The listing builds one solid part. Answer for the finished solid, in the listing's coordinates (mm). Round coordinates to 2 decimals unless told otherwise and drop trailing zeros. Write each loop counter-clockwise with the first axis right and the second up, starting at its lowest first coordinate (ties: lowest second). Pieces come first, ordered by that corner, then holes. Notation, with made-up numbers: M 69.5,33 L 114.5,33 A22 ccw 114.5,71 Z; hole C -28,7 d1. An arc over 180 degrees is marked long. One line per item, written item: value. Start each with the question number.
(1) Section B-B (x = 150.1) is taken. Determine the outline of the cut face in (y, z).
(2) Given P1, Ø3, axis at x = 87.5, z = -220, coming from the +Y side; P2, Ø1, axis at x = 38.5, y = 3, coming from the -Z side; P3, Ø1.9, axis at x = 34.5, z = 3, coming from the -Y side; P4, Ø4, axis at x = 17.53, z = -54.65, coming from the -Y side, each flat-ended and moving along its own axis, determine where each tip first touches the part or whether it passes through.
(3) Section A-A (z = -31) is taken. Determine the outline of the cut face in (x, y), plus the area to 3 significant figures.
(4) Section D-D (y = 2.5) is taken. State how many separate pieces and enclosed holes the cut face has, plus the area to 3 significant figures.
(5) Section C-C (z = -158.15) is taken. Determine the outline of the cut face in (x, y), plus the area to 3 significant figures.
(6) Consider probe 1 along Z at (x, y) = (167.15, 2.75); probe 2 along Z at (x, y) = (150.1, 2.75); probe 3 along Z at (x, y) = (147.5, 2.5). Determine where each line is inside the solid, lowest interval first.
```python
from build123d import *

# Parameters (mm, degrees)
SKETCH4_W           = 184.15
SKETCH4_H           = 215.9
BOSS_EXTRUDE2_DEPTH = 6.35
BOSS_EXTRUDE3_DEPTH = 6.35
BOSS_EXTRUDE4_DEPTH = 6.35
SKETCH7_W           = 5.08
SKETCH7_H           = 6.35
BOSS_EXTRUDE5_DEPTH = 3.81
SKETCH12_R          = 2.54
CUT_EXTRUDE4_DEPTH  = 7.35
SKETCH18_R          = 2.5
CUT_EXTRUDE8_DEPTH  = 10
SKETCH19_R          = 2.5
CUT_EXTRUDE9_DEPTH  = 10
SKETCH20_R          = 3
CUT_EXTRUDE10_DEPTH = 7.35
CUT_EXTRUDE11_DEPTH = 6.35
CUT_EXTRUDE12_DEPTH = 6.35
CUT_EXTRUDE13_DEPTH = 6.35
CUT_EXTRUDE14_DEPTH = 6.35
CUT_EXTRUDE15_DEPTH = 6.35


with BuildPart() as part:
    # Sketch4 → Boss-Extrude2 (new body)
    with BuildSketch(Plane(origin=(0, 0, 0), x_dir=(1, 0, 0), z_dir=(0, 1, 0))):
        with Locations((92.075, 107.95)):
            Rectangle(SKETCH4_W, SKETCH4_H)
    extrude(amount=BOSS_EXTRUDE2_DEPTH)

    # Sketch5 → Boss-Extrude3 (add)
    with BuildSketch(Plane.XY):
        with BuildLine():
            Line((15.875, 6.35), (66.675, 6.35))
            ThreePointArc((66.675, 6.35), (69.85, 3.175), (66.675, 0))
            Line((66.675, 0), (15.875, 0))
            ThreePointArc((15.875, 0), (12.7, 3.175), (15.875, 6.35))
        make_face()
    boss_extrude3 = extrude(amount=BOSS_EXTRUDE3_DEPTH)

    # Mirror1: Boss-Extrude3 across plane
    add(boss_extrude3.mirror(Plane(origin=(92.075, 0, 0), x_dir=(0, 0, 1), z_dir=(1, 0, 0))))

    # Sketch6 → Boss-Extrude4 (add)
    with BuildSketch(Plane(origin=(0, 0, -215.9), x_dir=(-1, 0, 0), z_dir=(0, 0, -1))):
        with BuildLine():
            Line((-117.475, 6.35), (-66.675, 6.35))
            ThreePointArc((-66.675, 6.35), (-63.5, 3.175), (-66.675, 0))
            Line((-66.675, 0), (-117.475, 0))
            ThreePointArc((-117.475, 0), (-120.65, 3.175), (-117.475, 6.35))
        make_face()
        with BuildLine():
            Line((-28.575, 6.35), (-3.175, 6.35))
            ThreePointArc((-3.175, 6.35), (0, 3.175), (-3.175, 0))
            Line((-3.175, 0), (-28.575, 0))
            ThreePointArc((-28.575, 0), (-31.75, 3.175), (-28.575, 6.35))
        make_face()
        with BuildLine():
            Line((-155.575, 6.35), (-180.975, 6.35))
            ThreePointArc((-180.975, 6.35), (-184.15, 3.175), (-180.975, 0))
            Line((-180.975, 0), (-155.575, 0))
            ThreePointArc((-155.575, 0), (-152.4, 3.175), (-155.575, 6.35))
        make_face()
    extrude(amount=BOSS_EXTRUDE4_DEPTH)

    # Sketch7 → Boss-Extrude5 (add)
    with BuildSketch(Plane(origin=(184.15, 0, 0), x_dir=(0, 0, -1), z_dir=(1, 0, 0))):
        with Locations((100.33, 3.175)):
            Rectangle(SKETCH7_W, SKETCH7_H)
    boss_extrude5 = extrude(amount=BOSS_EXTRUDE5_DEPTH)

    # Mirror3: Boss-Extrude5 across plane
    add(boss_extrude5.mirror(Plane.ZY.offset(-92.075)))

    # Sketch12 → Cut-Extrude4 (cut, through all)
    with BuildSketch(Plane.XZ):
        with Locations((17.528627724, -54.65)):
            Circle(SKETCH12_R)
        with Locations((167.15, -54.65)):
            Circle(SKETCH12_R)
        with Locations((167.15, -106.15)):
            Circle(SKETCH12_R)
        with Locations((17.528627724, -106.15)):
            Circle(SKETCH12_R)
        with Locations((17.528627724, -158.15)):
            Circle(SKETCH12_R)
        with Locations((167.15, -158.15)):
            Circle(SKETCH12_R)
    extrude(amount=-CUT_EXTRUDE4_DEPTH, mode=Mode.SUBTRACT)

    # Sketch18 → Cut-Extrude8 (cut)
    with BuildSketch(Plane(origin=(0, 6.35, 0), x_dir=(1, 0, 0), z_dir=(0, 1, 0))):
        with Locations((105.290220108, 49.015069715)):
            Circle(SKETCH18_R)
        with Locations((133.990220108, 49.015069715)):
            Circle(SKETCH18_R)
        with Locations((119.640220108, 96.915069715)):
            Circle(SKETCH18_R)
    extrude(amount=-CUT_EXTRUDE8_DEPTH, mode=Mode.SUBTRACT)

    # Sketch19 → Cut-Extrude9 (cut)
    with BuildSketch(Plane(origin=(0, 6.35, 0), x_dir=(1, 0, 0), z_dir=(0, 1, 0))):
        with Locations((75.754890742, 56.124247339)):
            Circle(SKETCH19_R)
        with Locations((38.754890742, 56.124247339)):
            Circle(SKETCH19_R)
        with Locations((75.754890742, 93.124247339)):
            Circle(SKETCH19_R)
        with Locations((38.754890742, 93.124247339)):
            Circle(SKETCH19_R)
    extrude(amount=-CUT_EXTRUDE9_DEPTH, mode=Mode.SUBTRACT)

    # Sketch20 → Cut-Extrude10 (cut, through all)
    with BuildSketch(Plane.XZ):
        with Locations((150.1, -182.048287602)):
            Circle(SKETCH20_R)
        with Locations((34.1, -182.048287602)):
            Circle(SKETCH20_R)
        with Locations((150.1, -31)):
            Circle(SKETCH20_R)
        with Locations((34.1, -31)):
            Circle(SKETCH20_R)
    extrude(amount=-CUT_EXTRUDE10_DEPTH, mode=Mode.SUBTRACT)

    # Sketch21 → Cut-Extrude11 (cut)
    with BuildSketch(Plane(origin=(0, 0, -222.25), x_dir=(-1, 0, 0), z_dir=(0, 0, -1))):
        with BuildLine():
            Line((-155.575, 6.35), (-180.975, 6.35))
            ThreePointArc((-180.975, 6.35), (-184.15, 3.175), (-180.975, 0))
            Line((-180.975, 0), (-155.575, 0))
            ThreePointArc((-155.575, 0), (-152.4, 3.175), (-155.575, 6.35))
        make_face()
        with BuildLine():
            Line((-155.575, 6.25), (-180.975, 6.25))
            ThreePointArc((-180.975, 6.25), (-184.05, 3.175), (-180.975, 0.1))
            Line((-180.975, 0.1), (-155.575, 0.1))
            ThreePointArc((-155.575, 0.1), (-152.5, 3.175), (-155.575, 6.25))
        make_face(mode=Mode.SUBTRACT)
    extrude(amount=-CUT_EXTRUDE11_DEPTH, mode=Mode.SUBTRACT)

    # Sketch22 → Cut-Extrude12 (cut)
    with BuildSketch(Plane(origin=(0, 0, -222.25), x_dir=(-1, 0, 0), z_dir=(0, 0, -1))):
        with BuildLine():
            Line((-66.675, 6.35), (-117.475, 6.35))
            ThreePointArc((-117.475, 6.35), (-120.65, 3.175), (-117.475, 0))
            Line((-117.475, 0), (-66.675, 0))
            ThreePointArc((-66.675, 0), (-63.5, 3.175), (-66.675, 6.35))
        make_face()
        with BuildLine():
            Line((-66.675, 6.25), (-117.475, 6.25))
            ThreePointArc((-117.475, 6.25), (-120.55, 3.175), (-117.475, 0.1))
            Line((-117.475, 0.1), (-66.675, 0.1))
            ThreePointArc((-66.675, 0.1), (-63.6, 3.175), (-66.675, 6.25))
        make_face(mode=Mode.SUBTRACT)
    extrude(amount=-CUT_EXTRUDE12_DEPTH, mode=Mode.SUBTRACT)

    # Sketch23 → Cut-Extrude13 (cut)
    with BuildSketch(Plane(origin=(0, 0, -222.25), x_dir=(-1, 0, 0), z_dir=(0, 0, -1))):
        with BuildLine():
            Line((-28.575, 0), (-3.175, 0))
            ThreePointArc((-3.175, 0), (0, 3.175), (-3.175, 6.35))
            Line((-3.175, 6.35), (-28.575, 6.35))
            ThreePointArc((-28.575, 6.35), (-31.75, 3.175), (-28.575, 0))
        make_face()
        with BuildLine():
            Line((-28.575, 0.1), (-3.175, 0.1))
            ThreePointArc((-3.175, 0.1), (-0.1, 3.175), (-3.175, 6.25))
            Line((-3.175, 6.25), (-28.575, 6.25))
            ThreePointArc((-28.575, 6.25), (-31.65, 3.175), (-28.575, 0.1))
        make_face(mode=Mode.SUBTRACT)
    extrude(amount=-CUT_EXTRUDE13_DEPTH, mode=Mode.SUBTRACT)

    # Sketch24 → Cut-Extrude14 (cut)
    with BuildSketch(Plane.XY.offset(6.35)):
        with BuildLine():
            Line((15.875, 0), (66.675, 0))
            ThreePointArc((66.675, 0), (69.85, 3.175), (66.675, 6.35))
            Line((66.675, 6.35), (15.875, 6.35))
            ThreePointArc((15.875, 6.35), (12.7, 3.175), (15.875, 0))
        make_face()
        with BuildLine():
            Line((15.875, 0.1), (66.675, 0.1))
            ThreePointArc((66.675, 0.1), (69.75, 3.175), (66.675, 6.25))
            Line((66.675, 6.25), (15.875, 6.25))
            ThreePointArc((15.875, 6.25), (12.8, 3.175), (15.875, 0.1))
        make_face(mode=Mode.SUBTRACT)
    extrude(amount=-CUT_EXTRUDE14_DEPTH, mode=Mode.SUBTRACT)

    # Sketch25 → Cut-Extrude15 (cut)
    with BuildSketch(Plane.XY.offset(6.35)):
        with BuildLine():
            Line((168.275, 6.35), (117.475, 6.35))
            ThreePointArc((117.475, 6.35), (114.3, 3.175), (117.475, 0))
            Line((117.475, 0), (168.275, 0))
            ThreePointArc((168.275, 0), (171.45, 3.175), (168.275, 6.35))
        make_face()
        with BuildLine():
            Line((168.275, 6.25), (117.475, 6.25))
            ThreePointArc((117.475, 6.25), (114.4, 3.175), (117.475, 0.1))
            Line((117.475, 0.1), (168.275, 0.1))
            ThreePointArc((168.275, 0.1), (171.35, 3.175), (168.275, 6.25))
        make_face(mode=Mode.SUBTRACT)
    extrude(amount=-CUT_EXTRUDE15_DEPTH, mode=Mode.SUBTRACT)


solid = part.part
```
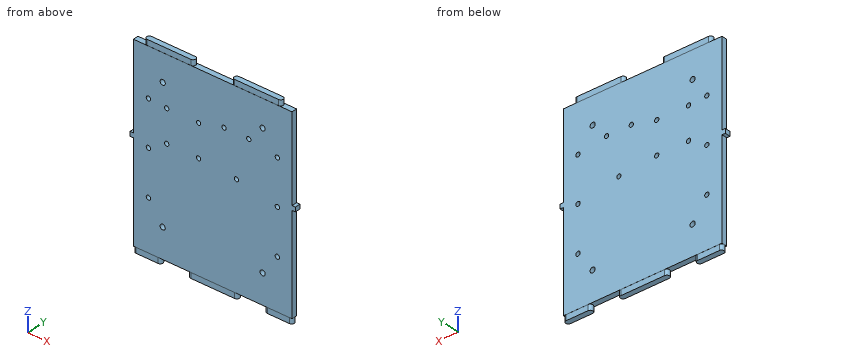
Recorded:
1. outline: M 0,-215.9 L 6.35,-215.9 L 6.35,-185.05 L 0,-185.05 Z; M 0,-179.05 L 6.35,-179.05 L 6.35,-34 L 0,-34 Z; M 0,-28 L 6.35,-28 L 6.35,0 L 6.25,0 L 6.25,6.35 L 0.1,6.35 L 0.1,0 L 0,0 Z
2. P1: stops at y = 6.25
2. P2: stops at z = -215.9
2. P3: stops at y = 0.1
2. P4: passes through
3. outline: M 0,0 L 31.1,0 L 31.1,6.35 L 0,6.35 Z; M 37.1,0 L 147.1,0 L 147.1,6.35 L 37.1,6.35 Z; M 153.1,0 L 184.15,0 L 184.15,6.35 L 153.1,6.35 Z
3. area: 1,090 mm2
4. separate pieces: 1
4. enclosed holes: 17
4. area: 40,900 mm2
5. outline: M 0,0 L 14.99,0 L 14.99,6.35 L 0,6.35 Z; M 20.07,0 L 164.61,0 L 164.61,6.35 L 20.07,6.35 Z; M 169.69,0 L 184.15,0 L 184.15,6.35 L 169.69,6.35 Z
5. area: 1,100 mm2
6. probe 1: z = -222.25 to -160.69, -155.61 to -108.69, -103.61 to -57.19, -52.11 to 6.35
6. probe 2: z = -215.9 to -185.05, -179.05 to -34, -28 to 6.35
6. probe 3: z = -215.9 to -183.54, -180.55 to -32.5, -29.5 to 6.35
